from build123d import *

# Parameters (mm, degrees)
CROQUIS1_R              = 25
CROQUIS1_R_2            = 11
SALIENTE_EXTRUIR1_DEPTH = 16.5
CROQUIS3_R              = 11
CROQUIS3_R_2            = 9.5
SALIENTE_EXTRUIR2_DEPTH = 10.5
SALIENTE_EXTRUIR3_START = -2
CROQUIS4_R              = 11
CROQUIS4_R_2            = 4
SALIENTE_EXTRUIR3_DEPTH = 2
SALIENTE_EXTRUIR4_START = -2.5
CROQUIS5_R              = 30
CROQUIS5_R_2            = 25
SALIENTE_EXTRUIR4_DEPTH = 2.5
CORTAR_EXTRUIR1_START   = 4
CROQUIS6_R              = 25
CROQUIS6_R_2            = 19
CORTAR_EXTRUIR1_DEPTH   = 4
SALIENTE_EXTRUIR5_REACH = 47.522
CROQUIS7_R              = 11
CROQUIS7_R_2            = 4.25
SALIENTE_EXTRUIR6_START = 2
CROQUIS8_R              = 6.1
CROQUIS8_R_2            = 4
SALIENTE_EXTRUIR6_DEPTH = 2
CROQUIS11_R             = 25
CROQUIS11_R_2           = 15
CORTAR_EXTRUIR2_DEPTH   = 1.5
CROQUIS13_R             = 4.25
CORTAR_EXTRUIR5_DEPTH   = 10
CORTAR_EXTRUIR6_START   = -10
CROQUIS14_R             = 4.25
CORTAR_EXTRUIR6_DEPTH   = 10


with BuildPart() as part:
    # Croquis1 → Saliente-Extruir1 (new body)
    with BuildSketch(Plane.XY):
        Circle(CROQUIS1_R)
        Circle(CROQUIS1_R_2, mode=Mode.SUBTRACT)
    extrude(amount=SALIENTE_EXTRUIR1_DEPTH)

    # Croquis3 → Saliente-Extruir2 (add, through all)
    with BuildSketch(Plane(origin=(0, 0, 6), x_dir=(-1, 0, 0), z_dir=(0, 0, -1))):
        Circle(CROQUIS3_R)
        Circle(CROQUIS3_R_2, mode=Mode.SUBTRACT)
    extrude(amount=-SALIENTE_EXTRUIR2_DEPTH)

    # Croquis4 → Saliente-Extruir3 (add)
    with BuildSketch(Plane.XY.offset(16.5).offset(SALIENTE_EXTRUIR3_START)):
        with Locations(Location((0, 0, 0), (0, 0, 180))):
            Circle(CROQUIS4_R)
        Circle(CROQUIS4_R_2, mode=Mode.SUBTRACT)
    extrude(amount=SALIENTE_EXTRUIR3_DEPTH)

    # Croquis5 → Saliente-Extruir4 (add)
    with BuildSketch(Plane.XY.offset(16.5).offset(SALIENTE_EXTRUIR4_START)):
        Circle(CROQUIS5_R)
        Circle(CROQUIS5_R_2, mode=Mode.SUBTRACT)
    extrude(amount=SALIENTE_EXTRUIR4_DEPTH)

    # Croquis6 → Cortar-Extruir1 (cut)
    with BuildSketch(Plane(origin=(0, 0, 11.75), x_dir=(-1, 0, 0), z_dir=(0, 0, -1)).offset(CORTAR_EXTRUIR1_START)):
        Circle(CROQUIS6_R)
        Circle(CROQUIS6_R_2, mode=Mode.SUBTRACT)
    extrude(amount=-CORTAR_EXTRUIR1_DEPTH, mode=Mode.SUBTRACT)

    # Croquis7 → Saliente-Extruir5 (add, up to next)
    with BuildSketch(Plane(origin=(0, 0, 0), x_dir=(-1, 0, 0), z_dir=(0, 0, -1)), mode=Mode.PRIVATE) as saliente_extruir5_sk1:
        Circle(CROQUIS7_R)
        Circle(CROQUIS7_R_2, mode=Mode.SUBTRACT)
    saliente_extruir5_tool1 = extrude(saliente_extruir5_sk1.sketch, amount=-SALIENTE_EXTRUIR5_REACH, mode=Mode.PRIVATE) - part.part
    add(saliente_extruir5_tool1.solids().sort_by_distance((10.688873, 0, 0))[0])

    # Croquis8 → Saliente-Extruir6 (add)
    with BuildSketch(Plane(origin=(0, 0, 0), x_dir=(-1, 0, 0), z_dir=(0, 0, -1)).offset(SALIENTE_EXTRUIR6_START)):
        with Locations(Location((0, 0, 0), (0, 0, 180))):
            Circle(CROQUIS8_R)
        with Locations(Location((0, 0, 0), (0, 0, 180))):
            Circle(CROQUIS8_R_2, mode=Mode.SUBTRACT)
    extrude(amount=-SALIENTE_EXTRUIR6_DEPTH)

    # Croquis11 → Cortar-Extruir2 (cut)
    with BuildSketch(Plane(origin=(0, 0, 0), x_dir=(-1, 0, 0), z_dir=(0, 0, -1))):
        Circle(CROQUIS11_R)
        Circle(CROQUIS11_R_2, mode=Mode.SUBTRACT)
    extrude(amount=-CORTAR_EXTRUIR2_DEPTH, mode=Mode.SUBTRACT)

    # Croquis13 → Cortar-Extruir5 (cut)
    with BuildSketch(Plane(origin=(0, 0, 14.5), x_dir=(-1, 0, 0), z_dir=(0, 0, -1))):
        Circle(CROQUIS13_R)
    extrude(amount=-CORTAR_EXTRUIR5_DEPTH, mode=Mode.SUBTRACT)

    # Croquis14 → Cortar-Extruir6 (cut)
    with BuildSketch(Plane.XY.offset(CORTAR_EXTRUIR6_START)):
        with Locations(Location((0, 0, 0), (0, 0, 180))):
            Circle(CROQUIS14_R)
    extrude(amount=CORTAR_EXTRUIR6_DEPTH, mode=Mode.SUBTRACT)


solid = part.part
Check sheet for the modelled part. Datum: model origin and axes. Units: mm. A direction names the side the tool comes from. Give positions to 0.01 mm unless a question says otherwise; leave off trailing zeros. Loops run counter-clockwise (first coordinate to the right, second up) from the corner with the lowest first, then second, coordinate; pieces in that order, holes last. Notation, with made-up numbers: M 2.5,7.25 L 38.5,7.25 A21 cw 38.5,37.25 Z; hole C 66.5,46 d2. An arc over 180 degrees is marked long. Return JSON: item names as keys, results as strings. Group by question number.
1. Tool access check on faces 5 (the cylindrical face through (-8.767, -16.856, 9.722)), 6 (the cylindrical face through (23.846, 7.509, 12.859)), 7 (the flat face through (6, 0, 16.5)). Record the directions out of +Z, -Z, +X, -X, +Y, -Y that give a thin tool (end or side, any length) a straight path to the whole face; none if there is none.
2. Cross-section at D-D on x = -10.5. Record the boundary of the cut face in (y, z).
3. Go/stop test with flat-tipped pins: pin 1 (10 mm diameter, centred on y = -6, z = 8, fed in from -X); pin 2 (1.5 mm diameter, centred on x = -2.5, z = 13.5, fed in from +Y); pin 3 (1.5 mm diameter, centred on y = 2, z = 2, fed in from +X). Record where each tip stops, or that it passes through.
4. Cross-section at A-A on y = 0. Record the boundary of the cut face in (x, z).
5. Thickness scan on L1, parallel to Y at x = 0, z = -1.35; L2, parallel to Y at x = 0, z = 13.25; L3, parallel to Z at x = -15, y = 17. Record the ranges inside material, lowest first.
6. Mould release check, pull along Z, two halves, no side actions. Record for faces 1 (the flat face through (4, 19, 7.75)), 2 (the flat face through (-6.5, 0.2, 0)), 3 (the flat face through (4, 19, 11.75)), 4 (the cylindrical face through (-29.97, 1.32, 15.23)): released by +Z, released by -Z, zero draft, split by the parting line, or undercut.
7. Cross-section at C-C on z = 9.25. Record the boundary of the cut face in (x, y), plus the area to 3 significant figures.
Return value:
{
 "1": {"face 5": "none", "face 6": "-Z", "face 7": "+Z, +X, -X, +Y, -Y"},
 "2": {"outline": "M -28.1,14 L -22.69,14 L -22.69,11.75 L -15.84,11.75 L -15.84,7.75 L -22.69,7.75 L -22.69,1.5 L -10.71,1.5 L -10.71,0 L 10.71,0 L 10.71,1.5 L 22.69,1.5 L 22.69,7.75 L 15.84,7.75 L 15.84,11.75 L 22.69,11.75 L 22.69,14 L 28.1,14 L 28.1,16.5 L -28.1,16.5 Z"},
 "3": {"pin 1": "x = -24.98", "pin 2": "y = 29.94", "pin 3": "x = 24.97"},
 "4": {"outline": "M -30,14 L -25,14 L -25,11.75 L -19,11.75 L -19,7.75 L -25,7.75 L -25,1.5 L -15,1.5 L -15,0 L -6.1,0 L -6.1,-2 L -4.25,-2 L -4.25,16.5 L -30,16.5 Z; M 4.25,-2 L 6.1,-2 L 6.1,0 L 15,0 L 15,1.5 L 25,1.5 L 25,7.75 L 19,7.75 L 19,11.75 L 25,11.75 L 25,14 L 30,14 L 30,16.5 L 4.25,16.5 Z"},
 "5": {"L1": "-6.1 to -4.25, 4.25 to 6.1", "L2": "-25 to -4.25, 4.25 to 25", "L3": "1.5 to 7.75, 11.75 to 16.5"},
 "6": {"face 1": "undercut", "face 2": "released by -Z", "face 3": "undercut", "face 4": "zero draft"},
 "7": {"outline": "C 0,0 d38; hole C 0,0 d8.5", "area": "1,080 mm^2"}
}
